Autodesk Inventor part; units mm, degrees
ref_plane "YZ Plane" through (0, 0, 0) normal (1, 0, 0) x (0, 1, 0)
ref_plane "XZ Plane" through (0, 0, 0) normal (0, 1, 0) x (-1, 0, 0)
ref_plane "XY Plane" through (0, 0, 0) normal (0, 0, 1) x (1, 0, 0)
sketch "Skizze1" plane through (0, 0, 0) normal (0, 0, 1) x (1, 0, 0)
  line L0 (-50, -25) -> (25, 25)
  line L1 (25, 25) -> (25, -25)
  line L2 (25, -25) -> (-50, -25)
  line L3 (0, 35) -> (0, -35)
  line L4 (-65, 0) -> (40, 0)
  line L5 (23, 21.263) -> (-43.3944, -23)
  line L6 (-43.3944, -23) -> (23, -23)
  line L7 (23, -23) -> (23, 21.263)
  line L8 (23, -23) -> (25, -23)
  line L9 (25, 22.5963) -> (23, 21.263)
  line L10 (-43.3944, -23) -> (-46.3944, -25)
  point P0 (0, 0)
  dimension "d0" = 50
  dimension "d1" = 75
  dimension "d2" = 25
  dimension "d3" = 25
  dimension "d4" = 2
extrude "Extrusion2" add sketch "Skizze1" along normal mid plane 200 contours L0 L4 L5 L10 L2 | L0 L3 L5 L4 | L0 L1 L9 L5 L3
sketch "Skizze2" plane through (0, 0, 100) normal (0, 0, 1) x (1, 0, 0)
  line L0 (-46.3944, -25) -> (25, 22.5963)
  line L1 (-46.3944, -25) -> (25, -25)
  line L2 (25, -25) -> (25, 22.5963)
  line L3 (25, 22.5963) -> (-46.3944, -25)
  line L4 (25, 25) -> (-50, -25)
  point P0 (0, 0)
extrude "Extrusion3" add sketch "Skizze2" against normal blind 2
sketch "Skizze3" plane through (0, 0, -100) normal (0, 0, -1) x (-1, 0, 0)
  line L0 (-25, 22.5963) -> (46.3944, -25)
  line L1 (46.3944, -25) -> (50, -25)
  line L2 (-25, 22.5963) -> (46.3944, -25)
  line L3 (46.3944, -25) -> (-25, -25)
  line L4 (-25, -25) -> (-25, 22.5963)
  line L5 (-25, -25) -> (-25, 25)
  point P0 (0, 0)
extrude "Extrusion4" add sketch "Skizze3" against normal blind 2
sketch "Skizze4" plane through (0, 0, 100) normal (0, 0, 1) x (1, 0, 0)
  circle A0 centre (15, 5) radius 1.6
  circle A1 centre (15, -10) radius 1.6
  line L0 (-50, -25) -> (25, -25)
  line L1 (25, -25) -> (25, 25)
  point P0 (0, 0)
  dimension "d13" = 3.2
  dimension "d14" = 3.2
  dimension "d15" = 15
  dimension "d16" = 15
  dimension "d17" = 10
  dimension "d18" = 10
extrude "Extrusion5" cut sketch "Skizze4" against normal up to surface (2 mm away)
sketch "Skizze5" plane through (0, 0, -100) normal (0, 0, -1) x (-1, 0, 0)
  circle A0 centre (-15, 5) radius 1.6
  circle A1 centre (-15, -10) radius 1.6
  line L0 (-25, 25) -> (-25, -25)
  line L1 (-25, -25) -> (50, -25)
  point P0 (0, 0)
  dimension "d21" = 3.2
  dimension "d22" = 3.2
  dimension "d23" = 10
  dimension "d24" = 10
  dimension "d25" = 15
  dimension "d26" = 15
extrude "Extrusion6" cut sketch "Skizze5" against normal up to surface (2 mm away)
properties part number "_3D-Druck"
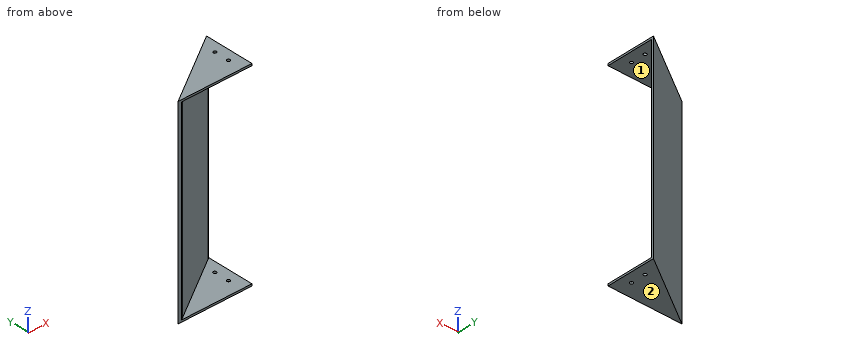
CAD build for the part. Positions are in the model's coordinates, mm. Face numbers are marked on the shaded views. A direction names the side the tool comes from. Give positions to 0.01 mm unless a question says otherwise; leave off trailing zeros. Order: outer loops, then holes, each group sorted by start corner. A loop starts at its lowest first (then second) coordinate and runs counter-clockwise, first axis right, second up. Notation, with made-up numbers: (48.5, 18) - (60.5, 18) arc R9 ccw to (60.5, 22) - close; hole circle Ø10 at (31, 5.5). An arc over 180 degrees is marked (long way). Write each question's results on one line, items separated by ' | '.
1. Probe L1, parallel to Z at x = 9, y = 7; L2, parallel to Y at x = 15, z = 98.9; L3, parallel to X at y = 13.5, z = -61. List the from-to ranges inside material, lowest first. Write a range as from..to.
Calculated:
L1: z = -100..-98, 98..100 | L2: y = -25..-11.6, -8.4..3.4, 6.6..18.33 | L3: x = 7.75..11.36
2. Saw through at A-A on y = -16. List the corners of the cut face in (x, z).
Calculated:
outline: (-36.5, -100) - (25, -100) - (25, -98) - (-32.89, -98) - (-32.89, 98) - (25, 98) - (25, 100) - (-36.5, 100) - close
3. 3-axis set-ups, long thin cutter, end or side, ignore diameter. For the marked faces 1 and 2: which of +Z, -Z, +X, -X, +Y, -Y reach the whole face in a straight line?
Calculated:
face 1: +X, -Y | face 2: -Z, +X, -X, +Y, -Y
4. Saw through at C-C on z = -10. List the corners of the cut face in (x, y), and give its area (3 significant figures).
Calculated:
outline: (-50, -25) - (-46.39, -25) - (-43.39, -23) - (23, 21.26) - (25, 22.6) - (25, 25) - close | area: 176 mm2
5. Saw through at B-B on x = -13.5. List the corners of the cut face in (y, z), and give its area (3 significant figures).
Calculated:
outline: (-25, -100) - (-0.67, -100) - (-0.67, 100) - (-25, 100) - (-25, 98) - (-3.07, 98) - (-3.07, -98) - (-25, -98) - close | area: 568 mm2
6. Pin check, flat tips, straight feed: pin 1 (1.5 mm diameter, centred on y = 16.5, z = 5, fed in from +X); pin 2 (1 mm diameter, centred on x = 7.5, y = 15, fed in from +Z); pin 3 (5 mm diameter, centred on y = -1, z = 49.5, fed in from +X); pin 4 (12 mm diameter, centred on y = 8, z = -8.5, fed in from -X). Stop position of each tip, or through.
Calculated:
pin 1: stops at x = 16.98 | pin 2: passes through | pin 3: stops at x = -6.64 | pin 4: stops at x = -9.5
